Answer from the drawing. Dimensions are ordinates in mm from the lowest x, y and z of the part. A direction names the side the tool comes from. Round coordinates to 2 decimals unless told otherwise and drop trailing zeros. Order: outer loops, then holes, each group sorted by start corner. A loop starts at its lowest first (then second) coordinate and runs counter-clockwise, first axis right, second up. Notation, with made-up numbers: (75.25, 81) - (98.25, 81) arc R26 ccw to (98.25, 111) - close; hole circle Ø2 at (-30, -35.75). An arc over 180 degrees is marked (long way). One line per question, with ' | ' between items. Start each with the question number.
1) The part is cut by section D-D, the plane x = 2. Give the vertices of the cut face in (y, z), plus the area to 4 significant figures.
2) Flat-ended cylindrical pins translate along their axes: pin 1 (2 mm diameter, centred on x = 3.5, y = 2, fed in from +Z); pin 2 (0.6 mm diameter, centred on y = 0, z = 2, fed in from -X); pin 3 (0.5 mm diameter, centred on y = 3, z = 1.5, fed in from +X). Find the tip coordinate at first contact, or state that the pin passes through.
3) The mould has two halves that part along X. Classify the marked faces 1, 2 and 3: pulls with the +X half, pulls with the -X half, needs draft (parallel to the pull), parting line crosses it, or undercut.
4) The part is cut by section B-B, the plane x = 4.25. Give the vertices of the cut face in (y, z).
5) Straight lines are drawn through the part: line 1 (X direction, y = 1, z = 3.9); line 2 (Z direction, x = 1.95, y = 0.65); line 3 (Y direction, x = 4.25, z = 2.6). For each, find the intervals that lie inside material, in ascending order. Write a range as from..to.
6) For the marked faces 4, 5, 6 and 7, determine the directions among +Z, -Z, +X, -X, +Y, -Y from which every point of the face is accessible in a straight line to the end or side of a thin tool.
7) The part is cut by section C-C, the plane z = 2.6. Give the vertices of the cut face in (x, y), plus the area to 3 significant figures.
8) The part is cut by section A-A, the plane y = 0.9. Give the vertices of the cut face in (x, z).
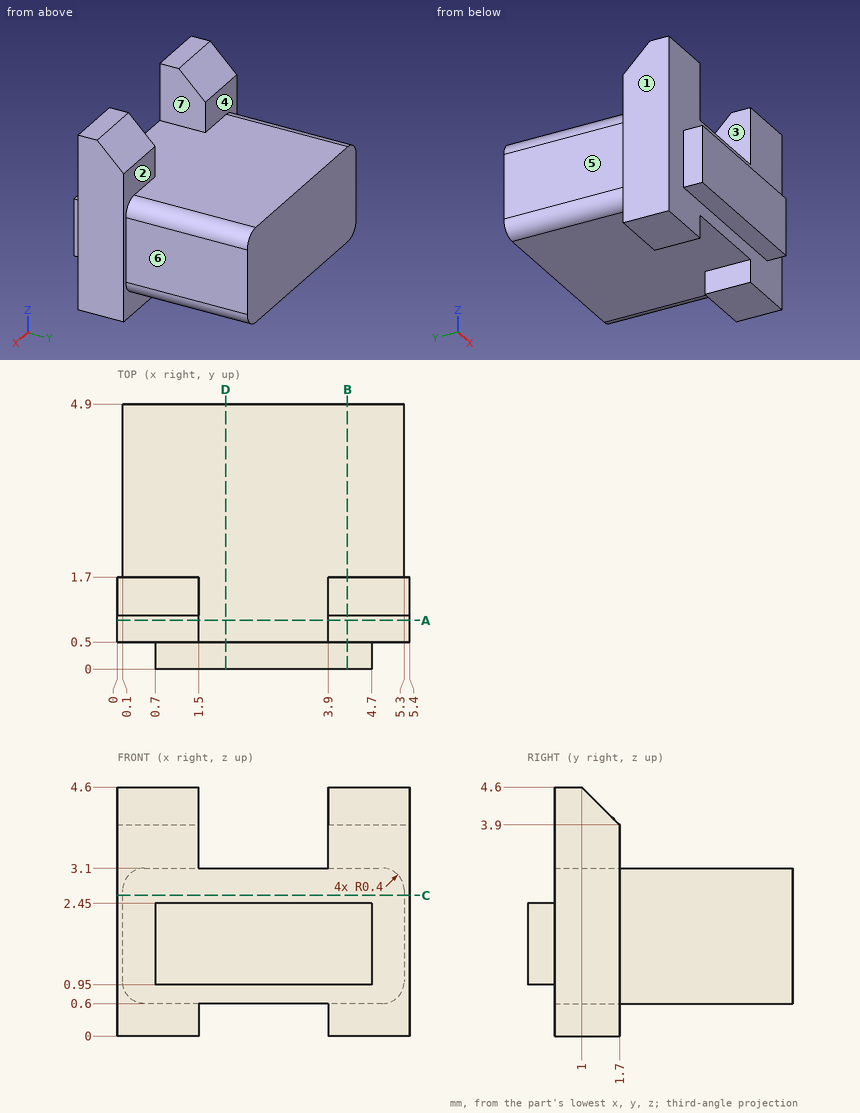
Values:
1) outline: (0, 0.95) - (0.5, 0.95) - (0.5, 0.6) - (4.9, 0.6) - (4.9, 3.1) - (0.5, 3.1) - (0.5, 2.45) - (0, 2.45) - close | area: 11.75 mm^2
2) pin 1: stops at z = 4.52 | pin 2: stops at x = 0.7 | pin 3: stops at x = 5.3
3) face 1: pulls with the -X half | face 2: needs draft | face 3: undercut
4) outline: (0, 0.95) - (0.5, 0.95) - (0.5, 0) - (1.7, 0) - (1.7, 0.6) - (4.9, 0.6) - (4.9, 3.1) - (1.7, 3.1) - (1.7, 3.9) - (1, 4.6) - (0.5, 4.6) - (0.5, 2.45) - (0, 2.45) - close
5) line 1: x = 0..1.5, 3.9..5.4 | line 2: z = 0.6..3.1 | line 3: y = 0.5..4.9
6) face 4: -X, +Y | face 5: +Z, -Z, -X, +Y | face 6: +Z, -Z, +X, +Y | face 7: +Z, +Y, -Y
7) outline: (0, 0.5) - (5.4, 0.5) - (5.4, 1.7) - (5.3, 1.7) - (5.3, 4.9) - (0.1, 4.9) - (0.1, 1.7) - (0, 1.7) - close | area: 23.1 mm^2
8) outline: (0, 0) - (1.5, 0) - (1.5, 0.6) - (3.9, 0.6) - (3.9, 0) - (5.4, 0) - (5.4, 4.6) - (3.9, 4.6) - (3.9, 3.1) - (1.5, 3.1) - (1.5, 4.6) - (0, 4.6) - close
